Read the model definition and answer for the solid it produces. Units are mm, in the model's axes. A direction names the side the tool comes from. Coordinates: 2 decimals unless noted, no trailing zeros. Loops run counter-clockwise (first coordinate to the right, second up) from the corner with the lowest first, then second, coordinate; pieces in that order, holes last. Notation, with made-up numbers: (51.25, 5) - (103.25, 5) arc R15 cw to (103.25, 15) - close; hole circle Ø7 at (83, 68). An arc over 180 degrees is marked (long way). Use CSV: the item, a comma, the result in double quotes.
```python
from build123d import *

# Parameters (mm, degrees)
F0_R     = 15.748
F0_R_2   = 1.27
F1_DEPTH = 1.6256
F2_W     = 13.6398
F2_H     = 9.46912
F3_DEPTH = 3.302
F4_W     = 21.336
F4_H     = 18.796
F5_DEPTH = 3.3528
F6_R     = 6.604


with BuildPart() as f1:
    # F0 (on Top) → F1 (new body)
    with BuildSketch(Plane.XY):
        Circle(F0_R)
        with Locations((-13.2461, 0)):
            Circle(F0_R_2, mode=Mode.SUBTRACT)
        with Locations((13.2461, 0)):
            Circle(F0_R_2, mode=Mode.SUBTRACT)
    extrude(amount=F1_DEPTH)

    # F2 (on face) → F3 (join)
    with BuildSketch(Plane.XY.offset(1.6256)):
        with Locations((1.2319, 0.00254)):
            Rectangle(F2_W, F2_H)
    extrude(amount=F3_DEPTH)

    # F4 (on Top) → F5 (join)
    with BuildSketch(Plane.XY):
        Rectangle(F4_W, F4_H)
    extrude(amount=-F5_DEPTH)

    # F6
    f6_edges = [f1.edges().sort_by_distance(p)[0] for p in [
        (10.668, -9.398, -1.6764),
        (-10.668, -9.398, -1.6764),
        (-10.668, 9.398, -1.6764),
        (10.668, 9.398, -1.6764),
    ]]
    fillet(f6_edges, radius=F6_R)


solid = f1.part
```
Q1. Find the intervals of material crossed by probe 1 along Y at (x, z) = (5, 3.5); probe 2 along Z at (x, y) = (-6.5, -13); probe 3 along Z at (x, y) = (5, 5.5), in increasing order. Write a range as [from, to].
Reported:
probe 1,"y = [-4.73, 4.74]"
probe 2,"z = [0, 1.63]"
probe 3,"z = [-3.35, 1.63]"
Q2. The part is cut by section A-A on y = 0. Determine the outline of the cut face in (x, z), and give its area (3 significant figures).
Reported:
outline,"(-15.75, 0) - (-14.52, 0) - (-14.52, 1.63) - (-15.75, 1.63) - close; (-11.98, 0) - (-10.67, 0) - (-10.67, -3.35) - (10.67, -3.35) - (10.67, 0) - (11.98, 0) - (11.98, 1.63) - (8.05, 1.63) - (8.05, 4.93) - (-5.59, 4.93) - (-5.59, 1.63) - (-11.98, 1.63) - close; (14.52, 0) - (15.75, 0) - (15.75, 1.63) - (14.52, 1.63) - close"
area,"160 mm²"
Q3. The part is cut by section D-D on z = 0.75. Determine the outline of the cut face in (x, y).
Reported:
outline,"circle Ø31.5 at (0, 0); hole circle Ø2.54 at (-13.25, 0); hole circle Ø2.54 at (13.25, 0)"
Q4. Given P1, Ø1, axis at x = 5, z = -1.5, coming from the -Y side; P2, Ø1.7, axis at y = -0.5, z = -2.5, coming from the -X side; P3, Ø1.7, axis at x = 1, z = 4, coming from the +Y side, each flat-ended and moving along its own axis, determine where each tip first touches the part or whether it passes through.
Reported:
P1,"stops at y = -9.38"
P2,"stops at x = -10.67"
P3,"stops at y = 4.74"
Q5. The part is cut by section C-C on x = 0. Determine the outline of the cut face in (y, z).
Reported:
outline,"(-15.75, 0) - (-9.4, 0) - (-9.4, -3.35) - (9.4, -3.35) - (9.4, 0) - (15.75, 0) - (15.75, 1.63) - (4.74, 1.63) - (4.74, 4.93) - (-4.73, 4.93) - (-4.73, 1.63) - (-15.75, 1.63) - close"
Q6. For a pull along Y with two mould halves and no side action, classify faces 1 (the face through (0, 9.398, -2)), 2 (the face through (-5.588, 0, 3)), 3 (the face through (11.977, 0.056, 0.801)), 4 (the face through (0, -9.398, -2)) as +Y half, -Y half, draft (parallel to the pull), parting line (faces both ways), or undercut.
Reported:
face 1,"+Y half"
face 2,"draft"
face 3,"undercut"
face 4,"-Y half"
Q7. The part is cut by section B-B on z = -1.25. Determine the outline of the cut face in (x, y), and give its area (3 significant figures).
Reported:
outline,"(-10.67, -2.79) arc R6.6 ccw to (-4.06, -9.4) - (4.06, -9.4) arc R6.6 ccw to (10.67, -2.79) - (10.67, 2.79) arc R6.6 ccw to (4.06, 9.4) - (-4.06, 9.4) arc R6.6 ccw to (-10.67, 2.79) - close"
area,"364 mm²"
Q8. A tool of negligible diameter and unlimited length cuts with its end or side. For faces 5 (the face through (-8.7, -7.5, -1.7)), 6 (the face through (1, 4.737, 3)), 7 (the face through (8.785, 7.412, -1.7)), 8 (the face through (8.052, 0, 3)), from which of +Z, -Z, +X, -X, +Y, -Y can it reach the whole face along a straight path? Write none if from no direction.
Reported:
face 5,"-Z, -X, -Y"
face 6,"+Z, +X, -X, +Y"
face 7,"-Z, +X, +Y"
face 8,"+Z, +X, +Y, -Y"
